The model under review builds one solid part; all positions refer to its coordinate system, in mm. Round coordinates to 2 decimals unless told otherwise and drop trailing zeros. Order: outer loops, then holes, each group sorted by start corner. A loop starts at its lowest first (then second) coordinate and runs counter-clockwise, first axis right, second up.
1) Consider section D-D (x = 86.5). Give the boundary of the cut face in (y, z).
2) Consider section C-C (y = 203). Give the boundary of the cut face in (x, z), then the cut area to 3 significant figures.
3) Consider section B-B (z = 3). Give the boundary of the cut face in (x, y).
4) Consider section A-A (x = 317.5). Give the boundary of the cut face in (y, z).
5) To check wall thickness, follow L1, parallel to Y at x = 317.5, z = 5.75; L2, parallel to Y at x = 312, z = 10; L3, parallel to X at y = 330, z = 2.75. State the ranges of each line that lie inside material, in increasing order.
6) Clearance check with flat-ended pins moving along their axes: P1, Ø6, axis at x = 121, y = 109.5, coming from the -Z side; P2, Ø6, axis at x = 74.5, z = 9.5, coming from the +Y side; P3, Ø3, axis at y = 190, z = 4.5, coming from the -X side; P4, Ø6, axis at y = 85.5, z = 8, coming from the -X side. State where each tip first meets the part, or that it passes through.
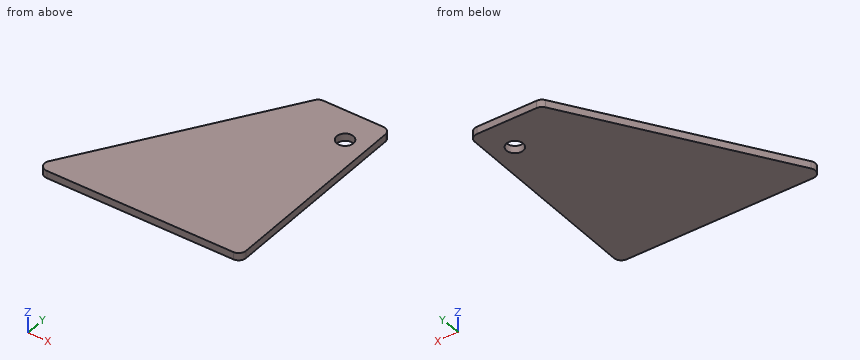
Autodesk Fusion 360 part; units mm, degrees
sketch "Sketch1" plane through (0, 0, 0) normal (0, 0, 1) x (1, 0, 0)
  line L0 (0, 0) -> (355.6, 0)
  line L1 (355.6, 0) -> (355.6, 355.6)
  line L2 (355.6, 355.6) -> (233.4623, 355.6)
  circle A0 centre (317.5, 300.4312) radius 14.2748
  line L3 (233.4623, 355.6) -> (0, 0)
  dimension "d1" = 355.6
  dimension "d3" = 28.5496
  dimension "d4" = 300.4312
  dimension "d5" = 38.1
extrude "Extrude1" add sketch "Sketch1" along normal blind 12.7
fillet "Fillet1" radius 12.7 4 edges at (355.6, 355.6, 6.35) (233.4623, 355.6, 6.35) (355.6, 0, 6.35) (0, 0, 6.35)
Answer below:
1. outline: (0, 0) - (131.75, 0) - (131.75, 12.7) - (0, 12.7) - close
2. outline: (133.28, 0) - (355.6, 0) - (355.6, 12.7) - (133.28, 12.7) - close
2. area: 2,820 mm2
3. outline: (12.91, 19.67) arc R12.7 ccw to (23.53, 0) - (342.9, 0) arc R12.7 ccw to (355.6, 12.7) - (355.6, 342.9) arc R12.7 ccw to (342.9, 355.6) - (240.32, 355.6) arc R12.7 ccw to (229.7, 349.87) - close; hole circle Ø28.55 at (317.5, 300.43)
4. outline: (0, 0) - (286.16, 0) - (286.16, 12.7) - (0, 12.7) - close; (314.71, 0) - (355.6, 0) - (355.6, 12.7) - (314.71, 12.7) - close
5. L1: y = 0 to 286.16, 314.71 to 355.6
5. L2: y = 0 to 287.26, 313.6 to 355.6
5. L3: x = 216.66 to 355.6
6. P1: stops at z = 0
6. P2: stops at y = 118.04
6. P3: stops at x = 123.76
6. P4: stops at x = 54.16
